Verification items for the finished model (mm, model axes). Face numbers are marked on the shaded views. A direction names the side the tool comes from. Coordinates: 2 decimals unless noted, no trailing zeros. Order: outer loops, then holes, each group sorted by start corner. A loop starts at its lowest first (then second) coordinate and runs counter-clockwise, first axis right, second up. Notation, with made-up numbers: M -12.75,72 L 4.25,72 A26 ccw 4.25,104 Z; hole C -22,19 d3. An arc over 180 degrees is marked long. Return JSON: item names as keys, results as strings.
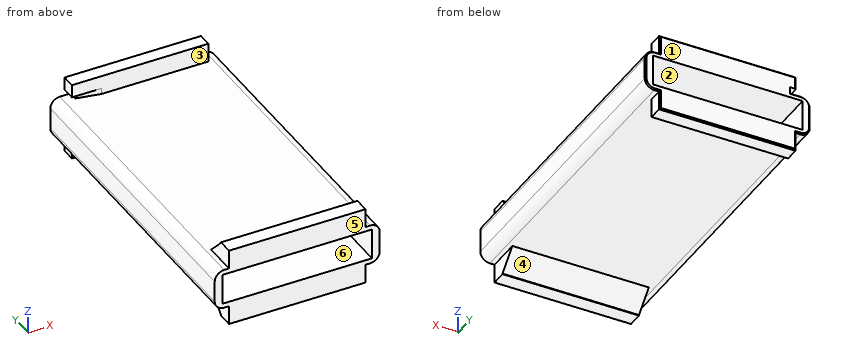
Autodesk Inventor part; units mm, degrees
ref_plane "YZ Plane" through (0, 0, 0) normal (1, 0, 0) x (0, 1, 0)
ref_plane "XZ Plane" through (0, 0, 0) normal (0, 1, 0) x (-1, 0, 0)
ref_plane "XY Plane" through (0, 0, 0) normal (0, 0, 1) x (1, 0, 0)
sketch "Skizze2" plane through (0, 0, 0) normal (0, 1, 0) x (-1, 0, 0)
  line L0 (-12.6, -2.6) -> (12.6, -2.6)
  line L1 (12.6, -2.6) -> (12.6, 2.6)
  line L2 (12.6, 2.6) -> (-12.6, 2.6)
  line L3 (-12.6, 2.6) -> (-12.6, -2.6)
  line L4 (-12.6, -2.6) -> (12.6, 2.6) construction
  line L5 (12.6, -2.6) -> (-12.6, 2.6) construction
  line L6 (-12.3, 3.4) -> (12.3, 3.4)
  line L7 (12.3, -3.4) -> (-12.3, -3.4)
  line L8 (-19.9239, 0) -> (19.9239, 0)
  line L9 (0, -5.2239) -> (0, 5.2239)
  arc A0 (-12.3, 3.4) -> (-13.9, 1.8) centre (-12.3, 1.8) ccw
  arc A1 (-13.9, -1.8) -> (-12.3, -3.4) centre (-12.3, -1.8) ccw
  arc A2 (13.9, 1.8) -> (12.3, 3.4) centre (12.3, 1.8) ccw
  arc A3 (12.3, -3.4) -> (13.9, -1.8) centre (12.3, -1.8) ccw
  line L10 (-13.9, 1.8) -> (-13.9, -1.8)
  line L11 (13.9, 1.8) -> (13.9, -1.8)
  point P0 (0, 0)
  dimension "d0" = 25.2
  dimension "d1" = 5.2
  dimension "d2" = 0.8
  dimension "d29" = 3.2
  dimension "d32" = 1.3
extrude "Extrusion1" add sketch "Skizze2" along normal blind 25.9 contours L0 L9 L7 A1 L10 L8 L3 | L0 L1 L8 L11 A3 L7 L9 | L8 L10 A0 L6 L9 L2 L3 | L1 L2 L9 L6 A2 L11 L8
sketch "Skizze3" plane through (0, 25.9, 0) normal (0, 1, 0) x (1, 0, 0)
  line L0 (12.6, 2.6) -> (12.6, -2.6)
  line L1 (12.6, -2.6) -> (-12.6, -2.6)
  line L2 (-12.6, -2.6) -> (-12.6, 2.6)
  line L3 (-12.6, 2.6) -> (12.6, 2.6)
  line L4 (12.3, 3.4) -> (-12.3, 3.4)
  line L5 (-12.3, -3.4) -> (12.3, -3.4)
  line L6 (19.46, 0) -> (-19.46, 0)
  line L7 (11.5, -3.4) -> (-11.5, -3.4)
  line L8 (-11.5, -3.4) -> (-11.5, -6.6)
  line L9 (-11.5, -6.6) -> (11.5, -6.6)
  line L10 (11.5, -6.6) -> (11.5, -3.4)
  line L11 (12.3, 3.4) -> (-12.3, 3.4)
  line L12 (11.5, 3.4) -> (-11.5, 3.4)
  line L13 (-11.5, 3.4) -> (-11.5, 6.6)
  line L14 (-11.5, 6.6) -> (11.5, 6.6)
  line L15 (11.5, 6.6) -> (11.5, 3.4)
  line L16 (0, 9.24) -> (0, -9.24)
  line L17 (-12.3, -3.4) -> (12.3, -3.4)
  arc A0 (12.3, -3.4) -> (13.9, -1.8) centre (12.3, -1.8) ccw
  arc A1 (13.9, 1.8) -> (12.3, 3.4) centre (12.3, 1.8) ccw
  arc A2 (-12.3, 3.4) -> (-13.9, 1.8) centre (-12.3, 1.8) ccw
  arc A3 (-13.9, -1.8) -> (-12.3, -3.4) centre (-12.3, -1.8) ccw
  line L18 (13.9, -1.8) -> (13.9, 1.8)
  line L19 (-13.9, 1.8) -> (-13.9, -1.8)
  dimension "d18" = 3.2
  dimension "d19" = 23
extrude "Extrusion2" add sketch "Skizze3" against normal blind 2.5 contours L16 L14 L15 L4 | L4 L13 L14 L16 | L16 L9 L8 L5 | L5 L10 L9 L16
mirror "Spiegeln1" about plane through (0, 0, 0) normal (0, 1, 0) of "Extrusion1", "Extrusion2"
chamfer "Fase1" distance 3.1 angle 45 2 edges at (0, -23.4, 3.4) (0, -23.4, -3.4)
sketch "Skizze7" plane through (0, 23.4, 0) normal (0, -1, 0) x (1, 0, 0)
  line L0 (13.4387, -2.2) -> (13.6, -2.2)
  line L1 (13.6, 1.5) -> (13.6, 2.2)
  line L2 (13.6, 2.2) -> (13.4387, 2.2)
  line L3 (11.5, 3.4) -> (11.5, 6.6)
  line L4 (11.5, 6.6) -> (-11.5, 6.6)
  line L5 (-11.5, 6.6) -> (-11.5, 3.4)
  line L6 (11.5, 3.4) -> (-11.5, 3.4)
  line L7 (-11.5, -3.4) -> (11.5, -3.4)
  line L8 (-11.5, -3.4) -> (-11.5, -6.6)
  line L9 (-11.5, -6.6) -> (11.5, -6.6)
  line L10 (11.5, -6.6) -> (11.5, -3.4)
  line L11 (-13.6, -2.2) -> (-13.4387, -2.2)
  line L12 (-13.4387, 2.2) -> (-13.6, 2.2)
  line L13 (-13.6, -1.5) -> (-13.6, -2.2)
  line L14 (-13.6, 2.2) -> (-13.6, 1.5)
  arc A0 (-13.6, -1.5) -> (-13.4387, -2.2) centre (-12, -1.5) ccw
  arc A1 (-13.4387, 2.2) -> (-13.6, 1.5) centre (-12, 1.5) ccw
  arc A2 (13.4387, -2.2) -> (13.6, -1.5) centre (12, -1.5) ccw
  line L15 (13.6, -2.2) -> (13.6, -1.5)
  arc A3 (13.6, 1.5) -> (13.4387, 2.2) centre (12, 1.5) ccw
extrude "Extrusion4" [suppressed]
chamfer "Fase2" [suppressed]
sketch "Skizze8" plane through (-11.5, 23.4, 3.4) normal (0, 0, 1) x (1, 0, 0)
  line L0 (0, 2.5) -> (23, 2.5)
  line L1 (0, 2.5) -> (0, 0)
  line L2 (23, 0) -> (0, 0)
  line L3 (23, 2.5) -> (23, 0)
  line L4 (0, 0) -> (23, 0)
  line L5 (0, 0) -> (0, 1)
  line L6 (0, 1) -> (5, 0)
  line L7 (5, 0) -> (0, 0)
  point P0 (11.5, -23.4)
  dimension "d33" = 1
  dimension "d34" = 5
extrude "Extrusion5" cut sketch "Skizze8" along normal blind 1 contours L6 L2 L1
sketch "Skizze9" plane through (-11.5, 25.9, 3.4) normal (-1, 0, 0) x (0, 0, 1)
  line L0 (0, -1.5) -> (1, -1.5)
  line L1 (1, -1.5) -> (1, -2.5)
  line L2 (3.2, -2.5) -> (1, -2.5)
  line L3 (3.2, 0) -> (3.2, -2.5)
  line L4 (0, 0) -> (3.2, 0)
  line L5 (0, -1.5) -> (0, 0)
  line L6 (1, -2.5) -> (0, -2.5)
  line L7 (0, -2.5) -> (0, 0)
  line L8 (0, 0) -> (1, 0)
  line L9 (1, 0) -> (1, -2.5)
  point P0 (-3.4, -25.9)
extrude "Extrusion6" cut sketch "Skizze9" against normal blind 1 contours L5 L4 L9 L0 | L0 L1 L6 L7
chamfer "Fase3" distance 0.2 angle 45 16 edges at (0, 25.9, 6.6) (11.5, 25.9, 5) (13.4314, 25.9, 2.9314) (13.9, 25.9, 0) (13.4314, 25.9, -2.9314) (11.9, 25.9, -3.4) (11.9, 25.9, 3.4) (11.5, 25.9, -5) (0, 25.9, -6.6) (-11.5, 25.9, -5) (-11.9, 25.9, -3.4) (-13.4314, 25.9, -2.9314) (-13.9, 25.9, 0) (-13.4314, 25.9, 2.9314) (-11.4, 25.9, 3.4) (-11.5, 25.9, 5.5)
properties part number "Spulenkoerper" material "PC/ABS-Kunststoff"
Q1. Material ranges on line 1 along X through (y, z) = (19, 2); line 2 along Z through (x, y) = (4, 18.5); line 3 along Y through (x, z) = (-8.25, 3.75), recorded low to high.
Values:
{"line 1": "-13.89 to -12.6, 12.6 to 13.89", "line 2": "-3.4 to -2.6, 2.6 to 3.4", "line 3": "-25.9 to -20.65, 23.75 to 25.9"}
Q2. Go/stop test with flat-tipped pins: pin 1 (3.5 mm diameter, centred on y = -22, z = 4.5, fed in from -X); pin 2 (7.5 mm diameter, centred on x = -5, y = 2, fed in from -Z); pin 3 (1.6 mm diameter, centred on y = -22.5, z = 5.5, fed in from +X). Record where each tip stops, or that it passes through.
Values:
{"pin 1": "x = -13.59", "pin 2": "z = -3.4", "pin 3": "x = 11.5"}
Q3. Cross-section at A-A, the plane z = 5.75. Record the boundary of the cut face in (x, y), and give its area (3 significant figures).
Values:
{"outline": "M -11.5,-25.9 L 11.5,-25.9 L 11.5,-22.65 L -11.5,-22.65 Z; M -11.5,23.4 L 11.5,23.4 L 11.5,25.7 L 11.3,25.9 L -11.3,25.9 L -11.5,25.7 Z", "area": "132 mm^2"}
Q4. Cross-section at C-C, the plane y = -22.5. Record the boundary of the cut face in (x, z).
Values:
{"outline": "M -13.9,-1.8 A1.6 ccw -12.3,-3.4 L -11.5,-3.4 L -11.5,-5.6 L 11.5,-5.6 L 11.5,-3.4 L 12.3,-3.4 A1.6 ccw 13.9,-1.8 L 13.9,1.8 A1.6 ccw 12.3,3.4 L 11.5,3.4 L 11.5,5.6 L -11.5,5.6 L -11.5,3.4 L -12.3,3.4 A1.6 ccw -13.9,1.8 Z; hole M -12.6,-2.6 L 12.6,-2.6 L 12.6,2.6 L -12.6,2.6 Z"}
Q5. Cross-section at B-B, the plane x = -10. Record the boundary of the cut face in (y, z).
Values:
{"outline": "M -25.9,-6.6 L -23.4,-6.6 L -23.4,-6.5 L -20.3,-3.4 L 23.4,-3.4 L 23.4,-6.6 L 25.7,-6.6 L 25.9,-6.4 L 25.9,-2.6 L -25.9,-2.6 Z; M -25.9,2.6 L 25.9,2.6 L 25.9,6.4 L 25.7,6.6 L 23.4,6.6 L 23.4,4.4 L 24.1,4.4 L 24.1,3.4 L -20.3,3.4 L -23.4,6.5 L -23.4,6.6 L -25.9,6.6 Z"}
Q6. Cross-section at D-D, the plane x = -5. Record the boundary of the cut face in (y, z).
Values:
{"outline": "M -25.9,-6.6 L -23.4,-6.6 L -23.4,-6.5 L -20.3,-3.4 L 23.4,-3.4 L 23.4,-6.6 L 25.7,-6.6 L 25.9,-6.4 L 25.9,-2.6 L -25.9,-2.6 Z; M -25.9,2.6 L 25.9,2.6 L 25.9,6.4 L 25.7,6.6 L 23.4,6.6 L 23.4,3.4 L -20.3,3.4 L -23.4,6.5 L -23.4,6.6 L -25.9,6.6 Z"}
Q7. Draft check along X on the marked faces 5 and 6. Enter one of: pulls with the +X half, pulls with the -X half, needs draft (parallel to the pull), parting line crosses it, or undercut.
Values:
{"face 5": "needs draft", "face 6": "undercut"}
Q8. Tool access check on the marked faces 1, 2, 3 and 4. Record the directions out of +Z, -Z, +X, -X, +Y, -Y that give a thin tool (end or side, any length) a straight path to the whole face; none if there is none.
Values:
{"face 1": "+Z, -Z, +X, -X, +Y", "face 2": "+Y, -Y", "face 3": "+Z, +X, -X", "face 4": "-Z, +X, -X"}
